from build123d import *

# Parameters (mm, degrees)
EXTRUDE_1_DEPTH     = 287.576527547
CUT_EXTRUDE_START   = -20
SKETCH_2_W          = 123.460031058
SKETCH_2_H          = 15.574638679
CUT_EXTRUDE_1_DEPTH = 277.47977873
SKETCH_3_W          = 53.30442173
SKETCH_3_H          = 30.05092592
CUT_EXTRUDE_2_DEPTH = 40
SKETCH_4_W          = 88.57938219
SKETCH_4_H          = 6.982300606
CUT_EXTRUDE_3_DEPTH = 296.966652169


with BuildPart() as part:
    # Эскиз1 → Вытянуть1 (new body)
    with BuildSketch(Plane(origin=(0, 0, 0), x_dir=(0, 0, -1), z_dir=(1, 0, 0))):
        Polygon((0, 0), (0, 60), (-4, 60), (-4, -5), (36, -5), (36, 0), align=None)
    extrude(amount=EXTRUDE_1_DEPTH)

    # Эскиз2 → Вырез-Вытянуть1 (cut, through all)
    with BuildSketch(Plane(origin=(0, 0, -36), x_dir=(-1, 0, 0), z_dir=(0, 0, -1)).offset(CUT_EXTRUDE_START)):
        with Locations((-128.492748506, -2.9676861)):
            Rectangle(SKETCH_2_W, SKETCH_2_H)
    extrude(amount=-CUT_EXTRUDE_1_DEPTH, mode=Mode.SUBTRACT)

    # Эскиз3 → Вырез-Вытянуть2 (cut)
    with BuildSketch(Plane(origin=(0, 0, 0), x_dir=(-1, 0, 0), z_dir=(0, 0, -1))):
        with Locations((-109.814559779, 49.461309937)):
            Rectangle(SKETCH_3_W, SKETCH_3_H)
    extrude(amount=-CUT_EXTRUDE_2_DEPTH, mode=Mode.SUBTRACT)

    # Эскиз4 → Вырез-Вытянуть3 (cut, through all)
    with BuildSketch(Plane(origin=(0, 0, 0), x_dir=(1, 0, 0), z_dir=(0, 1, 0))):
        with Locations((110.214944544, 33.390941069)):
            Rectangle(SKETCH_4_W, SKETCH_4_H)
    extrude(amount=-CUT_EXTRUDE_3_DEPTH, mode=Mode.SUBTRACT)


solid = part.part
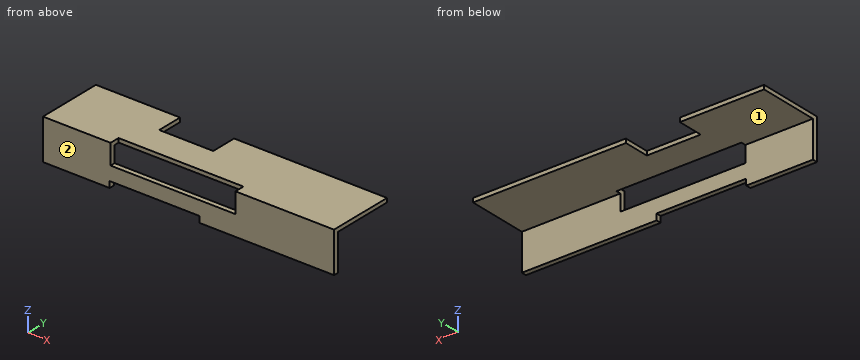
Geometry: final body of the model. Coordinates: model frame, mm. Face numbers are marked on the shaded views. A direction names the side the tool comes from. Give positions to 0.01 mm unless a question says otherwise; leave off trailing zeros. Write each loop counter-clockwise with the first axis right and the second up, starting at its lowest first coordinate (ties: lowest second). Pieces come first, ordered by that corner, then holes. Notation, with made-up numbers: (69, 88) - (95, 88) arc R22 ccw to (95, 106) - close; hole circle Ø8 at (32.25, 62). An arc over 180 degrees is marked (long way). Return JSON: item names as keys, results as strings. Group by question number.
1) Section C-C on x = 249.5. Return the cut outline in (y, z).
2) Section D-D on z = -26. Return the cut outline in (x, y).
3) Section B-B on y = 55. Return the cut outline in (x, z), plus the area to 3 significant figures.
4) First-contact query: P1, Ø1.5, axis at x = 38, y = 41.5, coming from the -Z side; P2, Ø4.5, axis at x = 103.5, z = 1.5, coming from the +Y side; P3, Ø1.5, axis at x = 94.5, y = -3, coming from the -Z side. Flat tips, straight axial feed; report the tip coordinate or a pass-through.
5) Line query: line 1 (Y direction, x = 24, z = -5.5); line 2 (Z direction, x = 65, y = 1). Output: solid intervals per line, ascending.
6) Section A-A on x = 132. Return the cut outline in (y, z).
7) Set-up query: the marked faces 1 and 2. Return all of +Z, -Z, +X, -X, +Y, -Y with unobstructed straight access to the full face (end or side cutting, diameter ignored); none if empty.
Filled in:
{
 "1": {"outline": "(-5, -36) - (0, -36) - (0, 0) - (60, 0) - (60, 4) - (-5, 4) - close"},
 "2": {"outline": "(0, -5) - (287.58, -5) - (287.58, 0) - (0, 0) - close"},
 "3": {"outline": "(0, 0) - (83.16, 0) - (83.16, 4) - (0, 4) - close; (136.47, 0) - (287.58, 0) - (287.58, 4) - (136.47, 4) - close", "area": "937 mm^2"},
 "4": {"P1": "stops at z = 0", "P2": "stops at y = 34.44", "P3": "stops at z = -29.9"},
 "5": {"line 1": "y = -5 to 0", "line 2": "z = 0 to 4"},
 "6": {"outline": "(-5, -29.9) - (0, -29.9) - (0, -16) - (-5, -16) - close; (4.82, 0) - (34.44, 0) - (34.44, 4) - (4.82, 4) - close"},
 "7": {"face 1": "-Z, +X, -X, +Y", "face 2": "+Z, -Z, +X, -X, -Y"}
}
